Could you check a few things on this model? Use its own coordinates, in mm. A direction names the side the tool comes from. Give positions to 0.01 mm unless a question says otherwise; leave off trailing zeros. Loops run counter-clockwise (first coordinate to the right, second up) from the corner with the lowest first, then second, coordinate; pieces in that order, holes last. Notation, with made-up numbers: (76.25, 86.5) - (94.25, 86.5) arc R7 ccw to (94.25, 99.5) - close; hole circle Ø4 at (15, 22.5). An arc over 180 degrees is marked (long way). Use CSV: the item, a comma, the result in double quotes.
Autodesk Inventor part; units mm, degrees
ref_plane "YZ Plane" through (0, 0, 0) normal (1, 0, 0) x (0, 1, 0)
ref_plane "XZ Plane" through (0, 0, 0) normal (0, 1, 0) x (-1, 0, 0)
ref_plane "XY Plane" through (0, 0, 0) normal (0, 0, 1) x (1, 0, 0)
sketch "Sketch1" plane through (0, 0, 0) normal (0, 1, 0) x (-1, 0, 0)
  circle A0 centre (0, 0) radius 0.8509
  dimension "d0" = 1.7018
extrude "Extrusion1" add sketch "Sketch1" along normal blind 4.699
sketch "Sketch2" plane through (0, 4.699, 0) normal (0, 1, 0) x (1, 0, 0)
  circle A0 centre (0, 0) radius 0.8509
  circle A1 centre (0, 0) radius 1.0795
  dimension "d3" = 2.159
extrude "Extrusion2" add sketch "Sketch2" along normal blind 0.8382 contours A0 | A1
sketch "Sketch3" plane through (0, 5.5372, 0) normal (0, 1, 0) x (1, 0, 0)
  circle A0 centre (0, 0) radius 1.0795
  circle A1 centre (0, 0) radius 0.5207
  dimension "d6" = 1.0414
extrude "Extrusion3" add sketch "Sketch3" along normal blind 8.255 contours A1
fillet "Fillet1" radius 0.508 1 edges at (-0.5207, 13.7922, 0)
properties part number "male_pin_component"
1) Suppose I cut it at B-B (y = 12). Please give me the cut outline in (x, z).
Answer below:
outline,"circle Ø1.04 at (0, 0)"
2) Which directions (+Z, -Z, +X, -X, +Y, -Y) give clear straight access to the entire face, cutting with the end or side of a thin tool? Please do faces 1 (the cylindrical face through (-0.786, 2.317, 0.326)), 2 (the flat face through (0, 0, 0)), 3 (the cylindrical face through (0.497, 9.356, 0.156)).
Answer below:
face 1,"-Y"
face 2,"+Z, -Z, +X, -X, -Y"
face 3,"+Y"
3) I'm going to push a flat-ended pin straight in: P1, Ø0.6, axis at x = -0.5, z = 0, coming from the +Y side. Where does the tip first touch, or does it pass through?
Answer below:
P1,"stops at y = 13.76"
4) Suppose I cut it at D-D (y = 3.25). Please give me the cut outline in (x, z), plus the area to 3 significant figures.
Answer below:
outline,"circle Ø1.7 at (0, 0)"
area,"2.27 mm2"
5) Suppose I cut it at C-C (z = 0.7). Please give me the cut outline in (x, y), plus the area to 3 significant figures.
Answer below:
outline,"(-0.82, 4.7) - (-0.48, 4.7) - (-0.48, 0) - (0.48, 0) - (0.48, 4.7) - (0.82, 4.7) - (0.82, 5.54) - (-0.82, 5.54) - close"
area,"5.92 mm2"
6) I need wall thicknesses on line 1 along X through (y, z) = (11.25, -0.05); line 2 along X through (y, z) = (6.25, -0.3); line 3 along Y through (x, z) = (0.8, -0.6). Which ranges of each line are inside material? Lowest first, please.
Answer below:
line 1,"x = -0.52 to 0.52"
line 2,"x = -0.43 to 0.43"
line 3,"y = 4.7 to 5.54"
7) Suppose I cut it at A-A (z = -0.65). Please give me the cut outline in (x, y).
Answer below:
outline,"(-0.86, 4.7) - (-0.55, 4.7) - (-0.55, 0) - (0.55, 0) - (0.55, 4.7) - (0.86, 4.7) - (0.86, 5.54) - (-0.86, 5.54) - close"
